```python
from build123d import *

# Parameters (mm, degrees)
SKETCH_R              = 15
PAD_DEPTH             = 98
SKETCH002_R           = 18
PAD002_DEPTH          = 3
SKETCH005_R           = 18
PAD004_DEPTH          = 3
SKETCH004_R           = 9.75
PAD005_DEPTH          = 2.5
SKETCH001_R           = 9.75
PAD006_DEPTH          = 2.5
SKETCH003_W           = 8
SKETCH003_H           = 10
POCKET_DEPTH          = 108
PAD007_DEPTH          = 1.5
PAD008_DEPTH          = 1.5
POLARPATTERN_COUNT    = 6
POLARPATTERN001_COUNT = 6


with BuildPart() as part:
    # Sketch → Pad (new body)
    with BuildSketch(Plane.XY):
        Circle(SKETCH_R)
    extrude(amount=PAD_DEPTH)

    # Sketch002 → Pad002 (join)
    with BuildSketch(Plane(origin=(0, 0, 0), x_dir=(1, 0, 0), z_dir=(0, 0, -1))):
        Circle(SKETCH002_R)
    extrude(amount=PAD002_DEPTH)

    # Sketch005 → Pad004 (join)
    with BuildSketch(Plane.XY.offset(98)):
        Circle(SKETCH005_R)
    extrude(amount=PAD004_DEPTH)

    # Sketch004 (on Face3 of Pad002) → Pad005 (join)
    with BuildSketch(Plane(origin=(0, 0, -3), x_dir=(1, 0, 0), z_dir=(0, 0, -1))):
        Circle(SKETCH004_R)
    extrude(amount=PAD005_DEPTH)

    # Sketch001 (on Face3 of Pad004) → Pad006 (join)
    with BuildSketch(Plane.XY.offset(101)):
        Circle(SKETCH001_R)
    extrude(amount=PAD006_DEPTH)

    # Sketch003 (on Face11 of Pad006) → Pocket (cut)
    with BuildSketch(Plane(origin=(0, 0, -5.5), x_dir=(1, 0, 0), z_dir=(0, 0, -1))):
        with Locations((14, 0)):
            Rectangle(SKETCH003_W, SKETCH003_H)
    extrude(amount=-POCKET_DEPTH, mode=Mode.SUBTRACT)

    # Sketch010 (on Face9 of Pocket) → Pad007 (join)
    with BuildSketch(Plane.XY):
        Polygon((-1.11579, 17.121659), (-0.012041, 17.758909), (1.091708, 17.121659), (1.091708, 15.84716), (-0.012041, 15.209911), (-1.11579, 15.84716), align=None)
    pad007 = extrude(amount=PAD007_DEPTH)

    # Sketch014 (on Face2 of Pad007) → Pad008 (join)
    with BuildSketch(Plane(origin=(0, 0, 98), x_dir=(1, 0, 0), z_dir=(0, 0, -1))):
        Polygon((-1.11579, 17.121659), (-0.012041, 17.758909), (1.091708, 17.121659), (1.091708, 15.84716), (-0.012041, 15.209911), (-1.11579, 15.84716), align=None)
    pad008 = extrude(amount=PAD008_DEPTH)

    # PolarPattern: Pad008 ×6 about axis
    polarpattern_axis = Axis((0, 0, 98), (0, 0, -1))
    for i in range(1, POLARPATTERN_COUNT):
        add(pad008.rotate(polarpattern_axis, i * 360 / POLARPATTERN_COUNT))

    # PolarPattern001: Pad007 ×6 about axis
    polarpattern001_axis = Axis((0, 0, 0), (0, 0, 1))
    for i in range(1, POLARPATTERN001_COUNT):
        add(pad007.rotate(polarpattern001_axis, i * 360 / POLARPATTERN001_COUNT))


solid = part.part
```
For this review, take the finished solid that the model builds, in its own axes (mm). A direction names the side the tool comes from. Coordinates: 2 decimals unless noted, no trailing zeros. Order: outer loops, then holes, each group sorted by start corner. A loop starts at its lowest first (then second) coordinate and runs counter-clockwise, first axis right, second up. Notation, with made-up numbers: (13.5, 32) - (51.5, 32) arc R18 cw to (51.5, 45) - close; hole circle Ø3 at (-19.5, 63.25). An arc over 180 degrees is marked (long way). Answer as a JSON object with one key per item and string values. Group by question number.
1. We need section D-D on y = -13.5. State the section outline as (x, z) points, then the cut area to 3 significant figures.
2. We need section C-C on z = 35. State the section outline as (x, y) points, then the cut area to 3 significant figures.
3. For faces 1 (the flat face through (14, 8, 96.5)), 2 (the flat face through (-8, -8, 101)), 3 (the flat face through (14, -8, 96.5)), 4 (the flat face through (-15, -3, 0)), list the 3-axis set-ups (+Z, -Z, +X, -X, +Y, -Y) from which the entire face can be reached by the end or side of a thin tool; tool diameter is ignored.
4. The part is to be moulded in two halves that separate along Y. For faces 5 (the flat face through (12, -5, 48)), 6 (the flat face through (-8, 8, -3)), 7 (the cylindrical face through (-17.986, -0.721, -1.479)), say which applies: pulls with the +Y half, pulls with the -Y half, needs draft (parallel to the pull), parting line crosses it, or undercut.
5. We need section B-B on x = 7. State the section outline as (y, z) points.
6. For probe 1 along Z at (x, y) = (5, -17); probe 2 along Y at (x, z) = (-0.5, 55); probe 3 along X at (y, z) = (-7.5, 76.5), list the stretches that pass through material, from the lowest coordinate up.
7. Clearance check with flat-ended pins moving along their axes: P1, Ø0.7, axis at x = -14.5, y = 8.5, coming from the +Z side; P2, Ø10, axis at x = -8.5, z = 82.5, coming from the -Y side; P3, Ø1.1, axis at x = 14.5, y = -8.5, coming from the -Z side. State where each tip first meets the part, or that it passes through.
8. We need section A-A on y = 0. State the section outline as (x, z) points, then the cut area to 3 significant figures.
Final values:
{
 "1": {"outline": "(-11.91, -3) - (11.91, -3) - (11.91, 0) - (6.54, 0) - (6.54, 98) - (11.91, 98) - (11.91, 101) - (-11.91, 101) - (-11.91, 98) - (-6.54, 98) - (-6.54, 0) - (-11.91, 0) - close", "area": "1,420 mm²"},
 "2": {"outline": "(10, -5) - (10, 5) - (14.14, 5) arc R15 ccw (long way) to (14.14, -5) - close", "area": "660 mm²"},
 "3": {"face 1": "+X, +Y", "face 2": "+Z", "face 3": "+X, -Y", "face 4": "none"},
 "4": {"face 5": "undercut", "face 6": "needs draft", "face 7": "parting line crosses it"},
 "5": {"outline": "(-16.58, -3) - (-6.79, -3) - (-6.79, -5.5) - (6.79, -5.5) - (6.79, -3) - (16.58, -3) - (16.58, 0) - (13.27, 0) - (13.27, 98) - (16.58, 98) - (16.58, 101) - (6.79, 101) - (6.79, 103.5) - (-6.79, 103.5) - (-6.79, 101) - (-16.58, 101) - (-16.58, 98) - (-13.27, 98) - (-13.27, 0) - (-16.58, 0) - close"},
 "6": {"probe 1": "-3 to 0, 98 to 101", "probe 2": "-14.99 to 14.99", "probe 3": "-12.99 to 12.99"},
 "7": {"P1": "z = 101", "P2": "y = -14.59", "P3": "z = -3"},
 "8": {"outline": "(-18, -3) - (-9.75, -3) - (-9.75, -5.5) - (9.75, -5.5) - (9.75, -3) - (10, -3) - (10, 101) - (9.75, 101) - (9.75, 103.5) - (-9.75, 103.5) - (-9.75, 101) - (-18, 101) - (-18, 98) - (-15, 98) - (-15, 0) - (-18, 0) - close", "area": "2,720 mm²"}
}
